Design review of the part shown in the three views and the two pictorial views. Dimensions are in mm from the part's minimum x, y and z. A direction names the side the tool comes from. Round coordinates to 2 decimals unless told otherwise and drop trailing zeros. Order: outer loops, then holes, each group sorted by start corner. A loop starts at its lowest first (then second) coordinate and runs counter-clockwise, first axis right, second up. Notation, with made-up numbers: M -37.5,55 L -6.5,55 A21 ccw -6.5,89 Z; hole C 11,48.25 d10. An arc over 180 degrees is marked long. Use a Markdown table: item, result. Add a question column.
(1) Take a section at D-D (x = 125). Write out the cut boundary in (y, z), then the cut area to 3 significant figures.
(2) Take a section at B-B (z = 125). Write out the cut boundary in (x, y).
(3) To check wall thickness, follow probe 1 along X at (y, z) = (70.5, 184.5); probe 2 along Y at (x, z) = (232, 64.5); probe 3 along X at (y, z) = (15, 125). State the ranges of each line that lie inside material, in increasing order. Write a range as from..to.
(4) For pin 1 (10 mm diameter, centred on x = 30, z = 189.5, fed in from +Y), flat-tipped, find the tip position at first contact; note if it passes through.
(5) Machinability: for the marked faces 4 and 5, which of the approach directions +Z, -Z, +X, -X, +Y, -Y give a long, thin tool a straight path to every point of the face, cutting with its end or side? Answer none if there is none.
(6) Take a section at A-A (x = 62). Write out the cut boundary in (y, z), then the cut area to 3 significant figures.
(7) The part is to be moulded in two halves that separate along Z. For the marked faces 1, 2 and 3, say which applies: released by +Z, released by -Z, zero draft, split by the parting line, or undercut.
(8) Take a section at C-C (y = 69). Write out the cut boundary in (x, z).
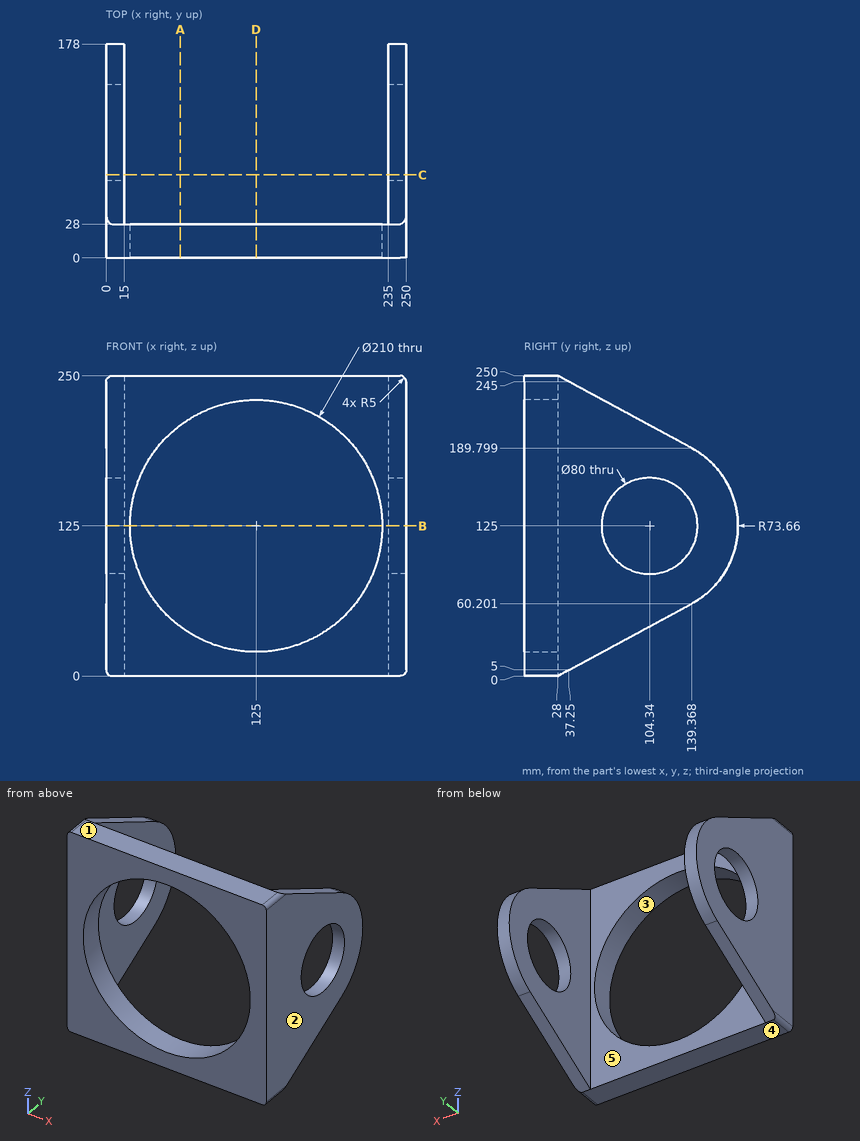
Verdict:
| question | item | result |
|---|---|---|
| 1 | outline | M 0,0 L 28,0 L 28,20 L 0,20 Z; M 0,230 L 28,230 L 28,250 L 0,250 Z |
| 1 | area | 1,120 mm^2 |
| 2 | outline | M 0,0 L 20,0 L 20,28 L 15,28 L 15,64.34 L 0,64.34 Z; M 0,144.34 L 15,144.34 L 15,178 L 0,178 Z; M 230,0 L 250,0 L 250,64.34 L 235,64.34 L 235,28 L 230,28 Z; M 235,144.34 L 250,144.34 L 250,178 L 235,178 Z |
| 3 | probe 1 | x = 0..15, 235..250 |
| 3 | probe 2 | y = 0..28 |
| 3 | probe 3 | x = 0..20, 230..250 |
| 4 | pin 1 | stops at y = 28 |
| 5 | face 4 | -Z, +X, -X, +Y, -Y |
| 5 | face 5 | +Z, -Z, +Y |
| 6 | outline | M 0,0 L 28,0 L 28,41 L 0,41 Z; M 0,209 L 28,209 L 28,250 L 0,250 Z |
| 6 | area | 2,300 mm^2 |
| 7 | face 1 | released by +Z |
| 7 | face 2 | zero draft |
| 7 | face 3 | undercut |
| 8 | outline | M 0,22.16 L 15,22.16 L 15,106.26 L 0,106.26 Z; M 0,143.74 L 15,143.74 L 15,227.84 L 0,227.84 Z; M 235,22.16 L 250,22.16 L 250,106.26 L 235,106.26 Z; M 235,143.74 L 250,143.74 L 250,227.84 L 235,227.84 Z |
